```python
from build123d import *

# Parameters (mm, degrees)
SKIZZE1_R                                            = 3
AUFSATZ_LINEAR_AUSTRAGEN1_DEPTH                      = 5
SKIZZE3_R                                            = 11.25
SCHNITT_LINEAR_AUSTRAGEN1_DEPTH                      = 2
STIRNSENKUNG_F_R_M3_ZYLINDERSCHRAUBE_MIT_D           = 3.4
STIRNSENKUNG_F_R_M3_ZYLINDERSCHRAUBE_MIT_CBORE_D     = 6.5
STIRNSENKUNG_F_R_M3_ZYLINDERSCHRAUBE_MIT_CBORE_DEPTH = 3.4
STIRNSENKUNG_F_R_M3_ZYLINDERSCHRAUBE_2_D             = 3.4
STIRNSENKUNG_F_R_M3_ZYLINDERSCHRAUBE_2_CBORE_D       = 6.5
STIRNSENKUNG_F_R_M3_ZYLINDERSCHRAUBE_2_CBORE_DEPTH   = 3.4
F_2_5_2_5_DURCHMESSER_BOHRUNG1_D                     = 2.5
F_2_5_2_5_DURCHMESSER_BOHRUNG1_DEPTH                 = 5


with BuildPart() as part:
    # Skizze1 → Aufsatz-Linear austragen1 (new body)
    with BuildSketch(Plane.XY):
        with BuildLine():
            Line((0, 0), (50, 0))
            Line((50, 0), (50, 55))
            ThreePointArc((50, 55), (45.606601718, 65.606601718), (35, 70))
            Line((35, 70), (15, 70))
            ThreePointArc((15, 70), (4.393398282, 65.606601718), (0, 55))
            Line((0, 55), (0, 0))
        make_face()
        with Locations((25, 45)):
            Circle(SKIZZE1_R, mode=Mode.SUBTRACT)
    extrude(amount=AUFSATZ_LINEAR_AUSTRAGEN1_DEPTH)

    # Skizze3 → Schnitt-Linear austragen1 (cut)
    with BuildSketch(Plane.XY.offset(5)):
        with Locations((25, 45)):
            Circle(SKIZZE3_R)
    extrude(amount=-SCHNITT_LINEAR_AUSTRAGEN1_DEPTH, mode=Mode.SUBTRACT)

    # Stirnsenkung f_r M3 Zylinderschraube mit (through all)
    with Locations(Plane(origin=(0, 0, 0), x_dir=(-1, 0, 0), z_dir=(0, 0, -1))):
        with Locations((-9.5, 29.5), (-9.5, 60.5), (-40.5, 60.5), (-40.5, 29.5)):
            CounterBoreHole(STIRNSENKUNG_F_R_M3_ZYLINDERSCHRAUBE_MIT_D / 2, STIRNSENKUNG_F_R_M3_ZYLINDERSCHRAUBE_MIT_CBORE_D / 2, STIRNSENKUNG_F_R_M3_ZYLINDERSCHRAUBE_MIT_CBORE_DEPTH)

    # Stirnsenkung f_r M3 Zylinderschraube 2 (through all)
    with Locations(Plane.XY.offset(5)):
        with Locations((38, 10), (12, 10)):
            CounterBoreHole(STIRNSENKUNG_F_R_M3_ZYLINDERSCHRAUBE_2_D / 2, STIRNSENKUNG_F_R_M3_ZYLINDERSCHRAUBE_2_CBORE_D / 2, STIRNSENKUNG_F_R_M3_ZYLINDERSCHRAUBE_2_CBORE_DEPTH)

    # Ø2.5 (2.5) Durchmesser Bohrung1
    with Locations(Plane(origin=(0, 0, 0), x_dir=(-1, 0, 0), z_dir=(0, 0, -1))):
        with Locations((-5, 20.4), (-5, 14)):
            Hole(F_2_5_2_5_DURCHMESSER_BOHRUNG1_D / 2, depth=F_2_5_2_5_DURCHMESSER_BOHRUNG1_DEPTH)


solid = part.part
```
The model under review builds one solid part; all positions refer to its coordinate system, in mm. A direction names the side the tool comes from. Round coordinates to 2 decimals unless told otherwise and drop trailing zeros. Order: outer loops, then holes, each group sorted by start corner. A loop starts at its lowest first (then second) coordinate and runs counter-clockwise, first axis right, second up. Notation, with made-up numbers: (85, 82.5) - (131, 82.5) arc R18 cw to (131, 98.5) - close; hole circle Ø7 at (65.5, 13.5). An arc over 180 degrees is marked (long way). Answer in a Markdown table with one row per item.
(1) For line 1 (Y direction, x = 38, z = 1.2); line 2 (Y direction, x = 40.5, z = 1.85); line 3 (Y direction, x = 9.5, z = 1.5), list the stretches that pass through material, from the lowest coordinate up. Write a range as from..to.
Result set:
| item | result |
|---|---|
| line 1 | y = 0..8.3, 11.7..27.42, 31.58..58.42, 62.58..69.7 |
| line 2 | y = 0..7.92, 12.08..26.25, 32.75..57.25, 63.75..68.96 |
| line 3 | y = 0..26.25, 32.75..57.25, 63.75..68.96 |
(2) Mouldability with a two-part tool opening along Y and no side actions: class faces 1 (the face through (25, 0, 2)), 2 (the face through (25, 35, 0)), 3 (the face through (39, 59, 3.4)) as released by +Y, released by -Y, zero draft, split by the parting line, or undercut.
Result set:
| item | result |
|---|---|
| face 1 | released by -Y |
| face 2 | zero draft |
| face 3 | undercut |
(3) Take a section at B-B on y = 14. Write out the cut boundary in (x, z).
Result set:
| item | result |
|---|---|
| outline | (0, 0) - (3.75, 0) - (3.75, 5) - (0, 5) - close; (6.25, 0) - (50, 0) - (50, 5) - (6.25, 5) - close |
(4) Machinability: for faces 4 (the face through (9.923, 63.722, 1.676)), 5 (the face through (41.1, 10.98, 3.32)), 6 (the face through (4.51, 65.72, 2.46)), which of the approach directions +Z, -Z, +X, -X, +Y, -Y give a long, thin tool a straight path to every point of the face, cutting with its end or side? Answer none if there is none.
Result set:
| item | result |
|---|---|
| face 4 | -Z |
| face 5 | +Z |
| face 6 | +Z, -Z, -X, +Y |
(5) Take a section at A-A on y = 29.5. Write out the cut boundary in (x, z), plus the area to 3 significant figures.
Result set:
| item | result |
|---|---|
| outline | (0, 0) - (6.25, 0) - (6.25, 3.4) - (7.8, 3.4) - (7.8, 5) - (0, 5) - close; (11.2, 3.4) - (12.75, 3.4) - (12.75, 0) - (37.25, 0) - (37.25, 3.4) - (38.8, 3.4) - (38.8, 5) - (11.2, 5) - close; (42.2, 3.4) - (43.75, 3.4) - (43.75, 0) - (50, 0) - (50, 5) - (42.2, 5) - close |
| area | 195 mm2 |
(6) Take a section at D-D on x = 17.5. Write out the cut boundary in (y, z), plus the area to 3 significant figures.
Result set:
| item | result |
|---|---|
| outline | (0, 0) - (70, 0) - (70, 5) - (53.39, 5) - (53.39, 3) - (36.61, 3) - (36.61, 5) - (0, 5) - close |
| area | 316 mm2 |
(7) Take a section at C-C on x = 24. Write out the cut boundary in (y, z).
Result set:
| item | result |
|---|---|
| outline | (0, 0) - (42.17, 0) - (42.17, 3) - (33.79, 3) - (33.79, 5) - (0, 5) - close; (47.83, 0) - (70, 0) - (70, 5) - (56.21, 5) - (56.21, 3) - (47.83, 3) - close |
(8) Clearance check with a flat-ended pin moving along its axis: P1, Ø2, axis at x = 12, y = 10, coming from the +Z side. State where the tip first meets the part, or that it passes through.
Result set:
| item | result |
|---|---|
| P1 | passes through |
